```python
from build123d import *

# Parameters (mm, degrees)
BOSS_EXTRUDE1_DEPTH        = 3
F_10_0MM_DOWEL_HOLE1_D     = 10
F_10_0MM_DOWEL_HOLE1_DEPTH = 3
F_3_0MM_DOWEL_HOLE1_D      = 3
F_3_0MM_DOWEL_HOLE1_DEPTH  = 3


with BuildPart() as part:
    # Sketch1 → Boss-Extrude1 (new body)
    with BuildSketch(Plane(origin=(0, 0, 0), x_dir=(1, 0, 0), z_dir=(0, 1, 0))):
        Polygon((0, 0), (139, 0), (109.720058283, 100), (29.279941717, 100), align=None)
    extrude(amount=BOSS_EXTRUDE1_DEPTH)

    # Ø10.0mm Dowel Hole1
    with Locations(Plane(origin=(0, 3, 0), x_dir=(1, 0, 0), z_dir=(0, 1, 0))):
        with Locations((69.5, 50)):
            Hole(F_10_0MM_DOWEL_HOLE1_D / 2, depth=F_10_0MM_DOWEL_HOLE1_DEPTH)

    # Ø3.0mm Dowel Hole1
    with Locations(Plane(origin=(0, 3, 0), x_dir=(1, 0, 0), z_dir=(0, 1, 0))):
        with Locations((59.55, 41.05), (59.55, 58.95), (79.45, 58.95), (79.45, 41.05)):
            Hole(F_3_0MM_DOWEL_HOLE1_D / 2, depth=F_3_0MM_DOWEL_HOLE1_DEPTH)


solid = part.part
```
The model under review builds one solid part; all positions refer to its coordinate system, in mm. Round coordinates to 2 decimals unless told otherwise and drop trailing zeros. Loops run counter-clockwise (first coordinate to the right, second up) from the corner with the lowest first, then second, coordinate; pieces in that order, holes last. Notation, with made-up numbers: (27, 60.25) - (50, 60.25) arc R12 cw to (50, 74.25) - close; hole circle Ø2 at (81, 77). An arc over 180 degrees is marked (long way). Use a Markdown table: item, result. Add a question column.
Q1. Add section A-A (x = 59.55). State the section outline as (y, z) points.
Q2. The part is to be moulded in two halves that separate along X. For faces 1 (the face through (14.845, 1.479, -50.7)), 2 (the face through (69, 1, 0)), 3 (the face through (60.66, 1.48, -42.06)), say which applies: pulls with the +X half, pulls with the -X half, needs draft (parallel to the pull), parting line crosses it, or undercut.
Q3. Add section D-D (z = -34). State the section outline as (x, y) points.
Q4. Add section C-C (z = -58.95). State the section outline as (x, y) points, plus the area to 3 significant figures.
Q5. Add section B-B (y = 1.7). State the section outline as (x, z) points.
Q6. For probe 1 along Z at (x, y) = (59.55, 2.1); probe 2 along X at (y, z) = (1.3, -50); probe 3 along X at (y, z) = (1, -49), list the stretches that pass through material, from the lowest coordinate up.
Worked answers:
| question | item | result |
|---|---|---|
| 1 | outline | (0, -100) - (3, -100) - (3, -60.45) - (0, -60.45) - close; (0, -57.45) - (3, -57.45) - (3, -42.55) - (0, -42.55) - close; (0, -39.55) - (3, -39.55) - (3, 0) - (0, 0) - close |
| 2 | face 1 | pulls with the -X half |
| 2 | face 2 | needs draft |
| 2 | face 3 | undercut |
| 3 | outline | (9.96, 0) - (129.04, 0) - (129.04, 3) - (9.96, 3) - close |
| 4 | outline | (17.26, 0) - (58.05, 0) - (58.05, 3) - (17.26, 3) - close; (61.05, 0) - (77.95, 0) - (77.95, 3) - (61.05, 3) - close; (80.95, 0) - (121.74, 0) - (121.74, 3) - (80.95, 3) - close |
| 4 | area | 295 mm² |
| 5 | outline | (0, 0) - (29.28, -100) - (109.72, -100) - (139, 0) - close; hole circle Ø3 at (59.55, -58.95); hole circle Ø3 at (59.55, -41.05); hole circle Ø10 at (69.5, -50); hole circle Ø3 at (79.45, -58.95); hole circle Ø3 at (79.45, -41.05) |
| 6 | probe 1 | -100 to -60.45, -57.45 to -42.55, -39.55 to 0 |
| 6 | probe 2 | 14.64 to 64.5, 74.5 to 124.36 |
| 6 | probe 3 | 14.35 to 64.6, 74.4 to 124.65 |
